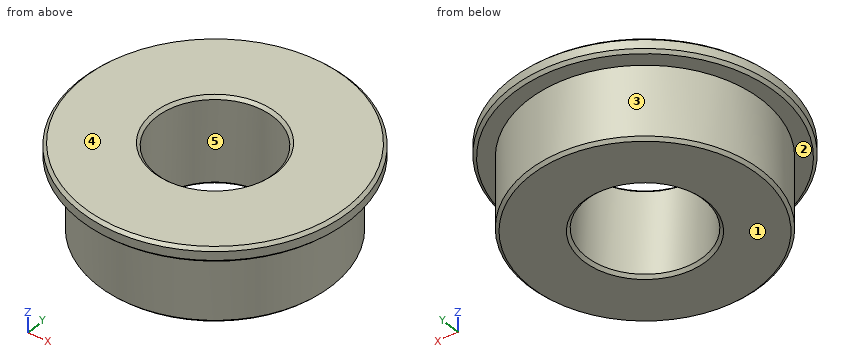
```python
from build123d import *

# Parameters (mm, degrees)
SKETCH_1_R      = 4
SKETCH_1_R_2    = 2
EXTRUDE_1_DEPTH = 3
EXTRUDE_START   = -0.5
SKETCH_2_R      = 4.6
SKETCH_2_R_2    = 4
EXTRUDE_2_DEPTH = 0.5
CHAMFER_1_SIZE  = 0.1


with BuildPart() as part:
    # 草图1 → 凸台-拉伸1 (new body)
    with BuildSketch(Plane.XY):
        Circle(SKETCH_1_R)
        Circle(SKETCH_1_R_2, mode=Mode.SUBTRACT)
    extrude(amount=EXTRUDE_1_DEPTH)

    # 草图2 → 凸台-拉伸2 (add)
    with BuildSketch(Plane.XY.offset(3).offset(EXTRUDE_START)):
        Circle(SKETCH_2_R)
        Circle(SKETCH_2_R_2, mode=Mode.SUBTRACT)
    extrude(amount=EXTRUDE_2_DEPTH)

    # 倒角1
    chamfer_1_edges = [part.edges().sort_by_distance(p)[0] for p in [
        (-4.6, 0, 2.5),
        (-4.6, 0, 3),
        (-4, 0, 0),
        (-2, 0, 0),
        (-2, 0, 3),
    ]]
    chamfer(chamfer_1_edges, length=CHAMFER_1_SIZE)


solid = part.part
```
Source: CAD feature listing. Evaluate the final solid. Frame: model axes, mm. Face numbers are marked on the shaded views. A direction names the side the tool comes from. Round coordinates to 2 decimals unless told otherwise and drop trailing zeros. Write each loop counter-clockwise with the first axis right and the second up, starting at its lowest first coordinate (ties: lowest second). Pieces come first, ordered by that corner, then holes. Notation, with made-up numbers: M 69.5,53 L 94.5,53 A4 cw 94.5,57 Z; hole C 39,85 d8. An arc over 180 degrees is marked long. Answer as a JSON object with one key per item and string values. Group by question number.
(1) Mould query, pull axis X, two halves, no side actions, for the marked faces 3, 4 and 5. Classes: +X half, -X half, draft (parallel to the pull), parting line (faces both ways), or undercut.
(2) Section query C-C on z = 2.75. Output: boundary loops of the cut face in (x, y), then the cut area to 3 significant figures.
(3) First-contact query: pin 1 (4 mm diameter, centred on x = -0.5, y = -1, fed in from -Z); pin 2 (1.5 mm diameter, centred on x = -2, z = 1.5, fed in from +Y); pin 3 (3 mm diameter, centred on x = 0, y = 0, fed in from -Z); pin 4 (1 mm diameter, centred on x = 0.5, z = 1.5, fed in from -Y). Flat tips, straight axial feed; report the tip coordinate or a pass-through.
(4) Ray query, line 1 (Y direction, x = 0, z = 1.4); line 2 (Z direction, x = -2.75, y = 3); line 3 (X direction, y = 0.75, z = 0.2). Return the intervals inside material, ascending. Write a range as [from, to].
(5) Section query A-A on y = 0. Output: boundary loops of the cut face in (x, z).
(6) Section query D-D on z = 2.1. Output: boundary loops of the cut face in (x, y).
(7) Reachability of the marked faces 1 and 2 from +Z, -Z, +X, -X, +Y, -Y: full face, straight path, thin tool, end or side. Return the list, or none.
Computed values:
{
 "1": {"face 3": "parting line", "face 4": "draft", "face 5": "undercut"},
 "2": {"outline": "C 0,0 d9.2; hole C 0,0 d4", "area": "53.9 mm^2"},
 "3": {"pin 1": "z = 0", "pin 2": "y = 3.8", "pin 3": "through", "pin 4": "y = -4"},
 "4": {"line 1": "[-4, -2], [2, 4]", "line 2": "[2.5, 3]", "line 3": "[-3.93, -1.85], [1.85, 3.93]"},
 "5": {"outline": "M -4.6,2.6 L -4.5,2.5 L -4,2.5 L -4,0.1 L -3.9,0 L -2.1,0 L -2,0.1 L -2,2.9 L -2.1,3 L -4.5,3 L -4.6,2.9 Z; M 2,0.1 L 2.1,0 L 3.9,0 L 4,0.1 L 4,2.5 L 4.5,2.5 L 4.6,2.6 L 4.6,2.9 L 4.5,3 L 2.1,3 L 2,2.9 Z"},
 "6": {"outline": "C 0,0 d8; hole C 0,0 d4"},
 "7": {"face 1": "-Z, +X, -X, +Y, -Y", "face 2": "-Z"}
}
